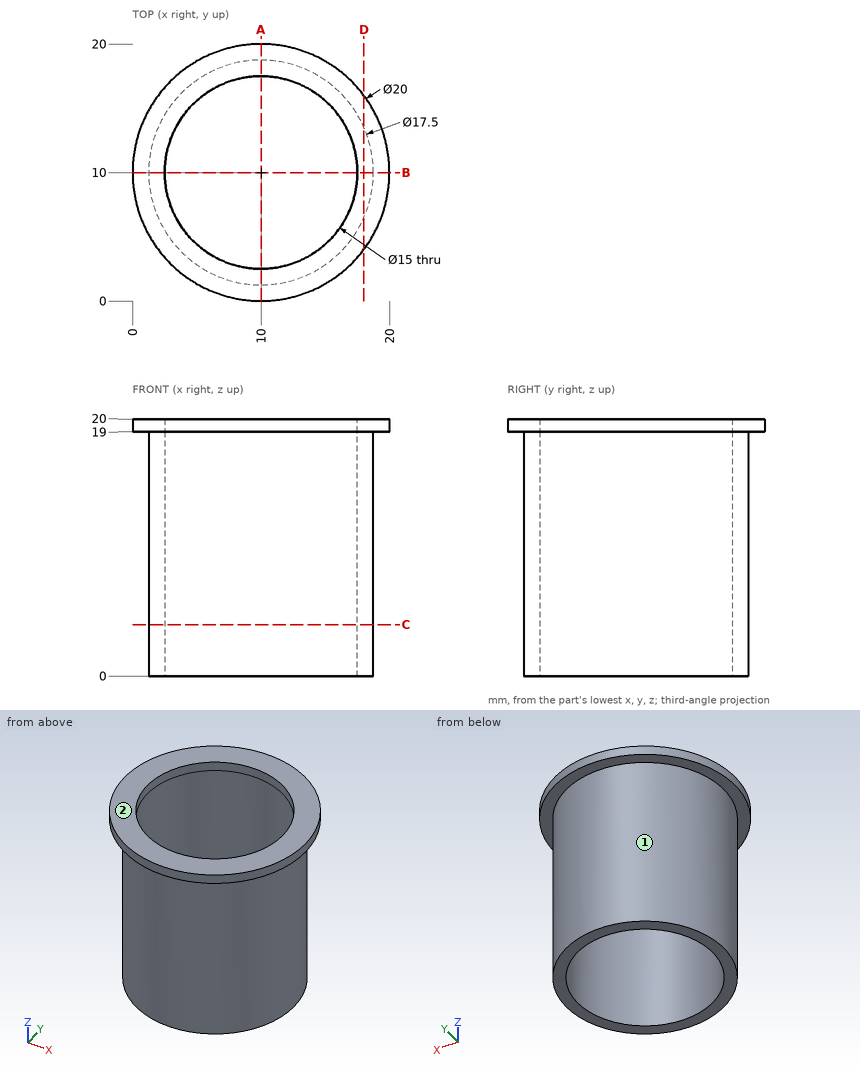
Part print with two shaded views. Sizes in mm from the minimum x, y, z corner. A direction names the side the tool comes from. Round coordinates to 2 decimals unless told otherwise and drop trailing zeros. Loops run counter-clockwise (first coordinate to the right, second up) from the corner with the lowest first, then second, coordinate; pieces in that order, holes last.
Item 1: Saw through at D-D (x = 18). List the corners of the cut face in (y, z).
Item 2: Saw through at C-C (z = 4). List the corners of the cut face in (x, y).
Item 3: Pin check, flat tips, straight feed: P1, Ø4, axis at y = 2.5, z = 17.5, coming from the +X side; P2, Ø2, axis at x = 3, y = 2.5, coming from the -Z side; P3, Ø6, axis at x = 12.5, z = 6, coming from the +Y side. Stop position of each tip, or through.
Item 4: Drill centre lines: line 1 along Y through (x, z) = (10, 19.2); line 2 along Z through (x, y) = (18.75, 9); line 3 along X through (y, z) = (15.75, 10.5). Where is each one in solid material? Low to high.
Item 5: Saw through at A-A (x = 10). List the corners of the cut face in (y, z), then the cut area to 3 significant figures.
Item 6: Which spindle directions (+Z, -Z, +X, -X, +Y, -Y) get a long thin tool onto all of the face, cutting with end or side? Do the marked faces 1 and 2. Say none if no direction does.
Worked answers:
1. outline: (4, 19) - (6.46, 19) - (6.46, 0) - (13.54, 0) - (13.54, 19) - (16, 19) - (16, 20) - (4, 20) - close
2. outline: circle Ø17.5 at (10, 10); hole circle Ø15 at (10, 10)
3. P1: stops at x = 17.86
3. P2: stops at z = 19
3. P3: stops at y = 18.75
4. line 1: y = 0 to 2.5, 17.5 to 20
4. line 2: z = 19 to 20
4. line 3: x = 3.4 to 5.18, 14.82 to 16.6
5. outline: (0, 19) - (1.25, 19) - (1.25, 0) - (2.5, 0) - (2.5, 20) - (0, 20) - close; (17.5, 0) - (18.75, 0) - (18.75, 19) - (20, 19) - (20, 20) - (17.5, 20) - close
5. area: 52.5 mm2
6. face 1: -Z
6. face 2: +Z, +X, -X, +Y, -Y
